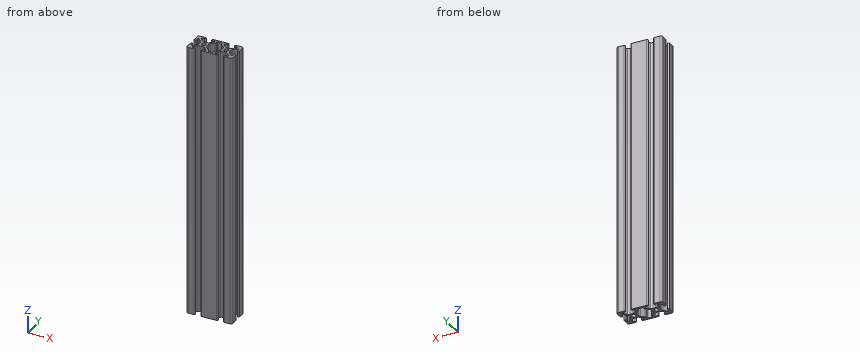
from build123d import *

# Parameters (mm, degrees)
SKETCH1_R      = 2.5
EXTRUDE1_DEPTH = 300


with BuildPart() as part:
    # Sketch1 → Extrude1 (new body)
    with BuildSketch(Plane.XY):
        with BuildLine():
            ThreePointArc((-10.5, 12.5), (-11.914213562, 11.914213562), (-12.5, 10.5))
            Line((-12.5, 10.5), (-12.5, 4.173306336))
            ThreePointArc((-12.5, 4.173306336), (-11.43, 3.103306336), (-10.36, 4.173306336))
            Line((-10.36, 4.173306336), (-10.36, 6.428177131))
            ThreePointArc((-10.36, 6.428177131), (-9.741558145, 7.353740775), (-8.649781387, 7.136572875))
            Line((-8.649781387, 7.136572875), (-5.328471504, 3.815262992))
            ThreePointArc((-5.328471504, 3.815262992), (-4.641301882, 2.786840976), (-4.4, 1.573734496))
            Line((-4.4, 1.573734496), (-4.4, -1.573734496))
            ThreePointArc((-4.4, -1.573734496), (-4.641301882, -2.786840976), (-5.328471504, -3.815262992))
            Line((-5.328471504, -3.815262992), (-8.649781387, -7.136572875))
            ThreePointArc((-8.649781387, -7.136572875), (-9.741558145, -7.353740775), (-10.36, -6.428177131))
            Line((-10.36, -6.428177131), (-10.36, -4.173306336))
            ThreePointArc((-10.36, -4.173306336), (-11.43, -3.103306336), (-12.5, -4.173306336))
            Line((-12.5, -4.173306336), (-12.5, -10.5))
            ThreePointArc((-12.5, -10.5), (-11.914213562, -11.914213562), (-10.5, -12.5))
            Line((-10.5, -12.5), (-4.173306336, -12.5))
            ThreePointArc((-4.173306336, -12.5), (-3.103306336, -11.43), (-4.173306336, -10.36))
            Line((-4.173306336, -10.36), (-6.428177131, -10.36))
            ThreePointArc((-6.428177131, -10.36), (-7.353740775, -9.741558145), (-7.136572875, -8.649781387))
            Line((-7.136572875, -8.649781387), (-3.815262992, -5.328471504))
            ThreePointArc((-3.815262992, -5.328471504), (-2.786840976, -4.641301882), (-1.573734496, -4.4))
            Line((-1.573734496, -4.4), (1.573734496, -4.4))
            ThreePointArc((1.573734496, -4.4), (2.786840976, -4.641301882), (3.815262992, -5.328471504))
            Line((3.815262992, -5.328471504), (7.136572875, -8.649781387))
            ThreePointArc((7.136572875, -8.649781387), (7.353740775, -9.741558145), (6.428177131, -10.36))
            Line((6.428177131, -10.36), (4.173306336, -10.36))
            ThreePointArc((4.173306336, -10.36), (3.103306336, -11.43), (4.173306336, -12.5))
            Line((4.173306336, -12.5), (20.826693664, -12.5))
            ThreePointArc((20.826693664, -12.5), (21.896693664, -11.43), (20.826693664, -10.36))
            Line((20.826693664, -10.36), (18.571822869, -10.36))
            ThreePointArc((18.571822869, -10.36), (17.646259225, -9.741558145), (17.863427125, -8.649781387))
            Line((17.863427125, -8.649781387), (21.184737008, -5.328471504))
            ThreePointArc((21.184737008, -5.328471504), (22.213159024, -4.641301882), (23.426265504, -4.4))
            Line((23.426265504, -4.4), (26.573734496, -4.4))
            ThreePointArc((26.573734496, -4.4), (27.786840976, -4.641301882), (28.815262992, -5.328471504))
            Line((28.815262992, -5.328471504), (32.136572875, -8.649781387))
            ThreePointArc((32.136572875, -8.649781387), (32.353740775, -9.741558145), (31.428177131, -10.36))
            Line((31.428177131, -10.36), (29.173306336, -10.36))
            ThreePointArc((29.173306336, -10.36), (28.103306336, -11.43), (29.173306336, -12.5))
            Line((29.173306336, -12.5), (35.5, -12.5))
            ThreePointArc((35.5, -12.5), (36.914213562, -11.914213562), (37.5, -10.5))
            Line((37.5, -10.5), (37.5, -4.173306336))
            ThreePointArc((37.5, -4.173306336), (36.43, -3.103306336), (35.36, -4.173306336))
            Line((35.36, -4.173306336), (35.36, -6.428177131))
            ThreePointArc((35.36, -6.428177131), (34.741558145, -7.353740775), (33.649781387, -7.136572875))
            Line((33.649781387, -7.136572875), (30.328471504, -3.815262992))
            ThreePointArc((30.328471504, -3.815262992), (29.641301882, -2.786840976), (29.4, -1.573734496))
            Line((29.4, -1.573734496), (29.4, 1.573734496))
            ThreePointArc((29.4, 1.573734496), (29.641301882, 2.786840976), (30.328471504, 3.815262992))
            Line((30.328471504, 3.815262992), (33.649781387, 7.136572875))
            ThreePointArc((33.649781387, 7.136572875), (34.741558145, 7.353740775), (35.36, 6.428177131))
            Line((35.36, 6.428177131), (35.36, 4.173306336))
            ThreePointArc((35.36, 4.173306336), (36.43, 3.103306336), (37.5, 4.173306336))
            Line((37.5, 4.173306336), (37.5, 10.5))
            ThreePointArc((37.5, 10.5), (36.914213562, 11.914213562), (35.5, 12.5))
            Line((35.5, 12.5), (29.173306336, 12.5))
            ThreePointArc((29.173306336, 12.5), (28.103306336, 11.43), (29.173306336, 10.36))
            Line((29.173306336, 10.36), (31.428177131, 10.36))
            ThreePointArc((31.428177131, 10.36), (32.353740775, 9.741558145), (32.136572875, 8.649781387))
            Line((32.136572875, 8.649781387), (28.815262992, 5.328471504))
            ThreePointArc((28.815262992, 5.328471504), (27.786840976, 4.641301882), (26.573734496, 4.4))
            Line((26.573734496, 4.4), (23.426265504, 4.4))
            ThreePointArc((23.426265504, 4.4), (22.213159024, 4.641301882), (21.184737008, 5.328471504))
            Line((21.184737008, 5.328471504), (17.863427125, 8.649781387))
            ThreePointArc((17.863427125, 8.649781387), (17.646259225, 9.741558145), (18.571822869, 10.36))
            Line((18.571822869, 10.36), (20.826693664, 10.36))
            ThreePointArc((20.826693664, 10.36), (21.896693664, 11.43), (20.826693664, 12.5))
            Line((20.826693664, 12.5), (4.173306336, 12.5))
            ThreePointArc((4.173306336, 12.5), (3.103306336, 11.43), (4.173306336, 10.36))
            Line((4.173306336, 10.36), (6.428177131, 10.36))
            ThreePointArc((6.428177131, 10.36), (7.353740775, 9.741558145), (7.136572875, 8.649781387))
            Line((7.136572875, 8.649781387), (3.815262992, 5.328471504))
            ThreePointArc((3.815262992, 5.328471504), (2.786840976, 4.641301882), (1.573734496, 4.4))
            Line((1.573734496, 4.4), (-1.573734496, 4.4))
            ThreePointArc((-1.573734496, 4.4), (-2.786840976, 4.641301882), (-3.815262992, 5.328471504))
            Line((-3.815262992, 5.328471504), (-7.136572875, 8.649781387))
            ThreePointArc((-7.136572875, 8.649781387), (-7.353740775, 9.741558145), (-6.428177131, 10.36))
            Line((-6.428177131, 10.36), (-4.173306336, 10.36))
            ThreePointArc((-4.173306336, 10.36), (-3.103306336, 11.43), (-4.173306336, 12.5))
            Line((-4.173306336, 12.5), (-10.5, 12.5))
        make_face()
        Circle(SKETCH1_R, mode=Mode.SUBTRACT)
        with BuildLine():
            Line((9.563960111, -9.552897559), (9.57, -9.358177131))
            ThreePointArc((9.57, -9.358177131), (9.330842974, -8.155853572), (8.649781387, -7.136572875))
            Line((8.649781387, -7.136572875), (5.328471504, -3.815262992))
            ThreePointArc((5.328471504, -3.815262992), (4.641301882, -2.786840976), (4.4, -1.573734496))
            Line((4.4, -1.573734496), (4.4, 1.573734496))
            ThreePointArc((4.4, 1.573734496), (4.641301882, 2.786840976), (5.328471504, 3.815262992))
            Line((5.328471504, 3.815262992), (8.649781387, 7.136572875))
            ThreePointArc((8.649781387, 7.136572875), (9.330842974, 8.155853572), (9.57, 9.358177131))
            Line((9.57, 9.358177131), (9.563229944, 9.576437453))
            ThreePointArc((9.563229944, 9.576437453), (9.777196412, 10.129004945), (10.322864597, 10.36))
            Line((10.322864597, 10.36), (14.677135403, 10.36))
            ThreePointArc((14.677135403, 10.36), (15.222803588, 10.129004945), (15.436770056, 9.576437453))
            Line((15.436770056, 9.576437453), (15.43, 9.358177131))
            ThreePointArc((15.43, 9.358177131), (15.669157026, 8.155853572), (16.350218613, 7.136572875))
            Line((16.350218613, 7.136572875), (19.671528496, 3.815262992))
            ThreePointArc((19.671528496, 3.815262992), (20.358698118, 2.786840976), (20.6, 1.573734496))
            Line((20.6, 1.573734496), (20.6, -1.573734496))
            ThreePointArc((20.6, -1.573734496), (20.358698118, -2.786840976), (19.671528496, -3.815262992))
            Line((19.671528496, -3.815262992), (16.350218613, -7.136572875))
            ThreePointArc((16.350218613, -7.136572875), (15.669157026, -8.155853572), (15.43, -9.358177131))
            Line((15.43, -9.358177131), (15.436770056, -9.576437453))
            ThreePointArc((15.436770056, -9.576437453), (15.222803588, -10.129004945), (14.677135403, -10.36))
            Line((14.677135403, -10.36), (10.322499075, -10.36))
            ThreePointArc((10.322499075, -10.36), (9.785097921, -10.137401154), (9.562499075, -9.6))
            ThreePointArc((9.562499075, -9.6), (9.562864421, -9.576437453), (9.563960111, -9.552897559))
        make_face(mode=Mode.SUBTRACT)
        with Locations((25, 0)):
            Circle(SKETCH1_R, mode=Mode.SUBTRACT)
    extrude(amount=-EXTRUDE1_DEPTH)


solid = part.part
CAD build for the part. Positions are in the model's coordinates, mm. Give positions to 0.01 mm unless a question says otherwise; leave off trailing zeros. Answer in a Markdown table with one row per item.
1. Flat gauge pins, fed straight in: pin 1 (3.5 mm diameter, centred on x = 25, z = -158.5, fed in from -Y); pin 2 (1.6 mm diameter, centred on y = 0.5, z = -106, fed in from +X); pin 3 (3 mm diameter, centred on x = 22, y = -2, fed in from +Z); pin 4 (2 mm diameter, centred on x = 26.5, z = -107, fed in from +Y). Where does each tip first touch, or does it go through?
Data:
| item | result |
|---|---|
| pin 1 | stops at y = -4.4 |
| pin 2 | stops at x = 29.4 |
| pin 3 | stops at z = 0 |
| pin 4 | stops at y = 4.54 |
2. Saw through at A-A, the plane z = -236. Count the separate pieces of the cut face and the enclosed holes in it, plus the area to 3 significant figures.
Data:
| item | result |
|---|---|
| separate pieces | 1 |
| enclosed holes | 3 |
| area | 486 mm² |
3. Probe probe 1 along X at (y, z) = (11, -43.5); probe 2 along X at (y, z) = (-9, -16); probe 3 along X at (y, z) = (6.25, -104). List the from-to ranges inside material, lowest first. Write a range as [from, to].
Data:
| item | result |
|---|---|
| probe 1 | x = [-12.44, -3.19], [3.19, 21.81], [28.19, 37.44] |
| probe 2 | x = [-12.5, -7.36], [7.36, 9.55], [15.45, 17.64], [32.36, 37.5] |
| probe 3 | x = [-12.5, -10.36], [-7.76, -4.74], [4.74, 7.76], [17.24, 20.26], [29.74, 32.76], [35.36, 37.5] |
